```python
from build123d import *

# Parameters (mm, degrees)
BOSS_EXTRUDE1_DEPTH = 428


with BuildPart() as part:
    # Sketch1 → Boss-Extrude1 (new body)
    with BuildSketch(Plane(origin=(0, 0, 0), x_dir=(0, 0, -1), z_dir=(1, 0, 0))):
        with BuildLine():
            Line((-12.5, 11.5), (-12.5, 3))
            Line((-12.5, 3), (-10.5, 3))
            Line((-10.5, 3), (-10.5, 6))
            Line((-10.5, 6), (-9.535533906, 6))
            Line((-9.535533906, 6), (-6.5, 2.964466094))
            Line((-6.5, 2.964466094), (-6.5, -2.964466094))
            Line((-6.5, -2.964466094), (-9.535533906, -6))
            Line((-9.535533906, -6), (-10.5, -6))
            Line((-10.5, -6), (-10.5, -3))
            Line((-10.5, -3), (-12.5, -3))
            Line((-12.5, -3), (-12.5, -11.5))
            ThreePointArc((-12.5, -11.5), (-12.207106781, -12.207106781), (-11.5, -12.5))
            Line((-11.5, -12.5), (-3, -12.5))
            Line((-3, -12.5), (-3, -10.5))
            Line((-3, -10.5), (-6, -10.5))
            Line((-6, -10.5), (-6, -9.535533906))
            Line((-6, -9.535533906), (-2.964466094, -6.5))
            Line((-2.964466094, -6.5), (2.964466094, -6.5))
            Line((2.964466094, -6.5), (6, -9.535533906))
            Line((6, -9.535533906), (6, -10.5))
            Line((6, -10.5), (3, -10.5))
            Line((3, -10.5), (3, -12.5))
            Line((3, -12.5), (11.5, -12.5))
            ThreePointArc((11.5, -12.5), (12.207106781, -12.207106781), (12.5, -11.5))
            Line((12.5, -11.5), (12.5, -3))
            Line((12.5, -3), (10.5, -3))
            Line((10.5, -3), (10.5, -6))
            Line((10.5, -6), (9.535533906, -6))
            Line((9.535533906, -6), (6.5, -2.964466094))
            Line((6.5, -2.964466094), (6.5, 2.964466094))
            Line((6.5, 2.964466094), (9.535533906, 6))
            Line((9.535533906, 6), (10.5, 6))
            Line((10.5, 6), (10.5, 3))
            Line((10.5, 3), (12.5, 3))
            Line((12.5, 3), (12.5, 11.5))
            ThreePointArc((12.5, 11.5), (12.207106781, 12.207106781), (11.5, 12.5))
            Line((11.5, 12.5), (3, 12.5))
            Line((3, 12.5), (3, 10.5))
            Line((3, 10.5), (6, 10.5))
            Line((6, 10.5), (6, 9.535533906))
            Line((6, 9.535533906), (2.964466094, 6.5))
            Line((2.964466094, 6.5), (-2.964466094, 6.5))
            Line((-2.964466094, 6.5), (-6, 9.535533906))
            Line((-6, 9.535533906), (-6, 10.5))
            Line((-6, 10.5), (-3, 10.5))
            Line((-3, 10.5), (-3, 12.5))
            Line((-3, 12.5), (-11.5, 12.5))
            ThreePointArc((-11.5, 12.5), (-12.207106781, 12.207106781), (-12.5, 11.5))
        make_face()
        with BuildLine():
            Line((-3.087755464, -1.885673936), (-3.585519377, -2.383437849))
            ThreePointArc((-3.585519377, -2.383437849), (-4.599238816, -4.599238816), (-2.383437849, -3.585519377))
            Line((-2.383437849, -3.585519377), (-1.885673936, -3.087755464))
            ThreePointArc((-1.885673936, -3.087755464), (-1.720751743, -3.0036254), (-1.537849315, -3.032329053))
            ThreePointArc((-1.537849315, -3.032329053), (0, -3.4), (1.537849315, -3.032329053))
            ThreePointArc((1.537849315, -3.032329053), (1.720751743, -3.0036254), (1.885673936, -3.087755464))
            Line((1.885673936, -3.087755464), (2.383437849, -3.585519377))
            ThreePointArc((2.383437849, -3.585519377), (4.599238816, -4.599238816), (3.585519377, -2.383437849))
            Line((3.585519377, -2.383437849), (3.087755464, -1.885673936))
            ThreePointArc((3.087755464, -1.885673936), (3.0036254, -1.720751743), (3.032329053, -1.537849315))
            ThreePointArc((3.032329053, -1.537849315), (3.4, 0), (3.032329053, 1.537849315))
            ThreePointArc((3.032329053, 1.537849315), (3.0036254, 1.720751743), (3.087755464, 1.885673936))
            Line((3.087755464, 1.885673936), (3.585519377, 2.383437849))
            ThreePointArc((3.585519377, 2.383437849), (4.599238816, 4.599238816), (2.383437849, 3.585519377))
            Line((2.383437849, 3.585519377), (1.885673936, 3.087755464))
            ThreePointArc((1.885673936, 3.087755464), (1.720751743, 3.0036254), (1.537849315, 3.032329053))
            ThreePointArc((1.537849315, 3.032329053), (0, 3.4), (-1.537849315, 3.032329053))
            ThreePointArc((-1.537849315, 3.032329053), (-1.720751743, 3.0036254), (-1.885673936, 3.087755464))
            Line((-1.885673936, 3.087755464), (-2.383437849, 3.585519377))
            ThreePointArc((-2.383437849, 3.585519377), (-4.599238816, 4.599238816), (-3.585519377, 2.383437849))
            Line((-3.585519377, 2.383437849), (-3.087755464, 1.885673936))
            ThreePointArc((-3.087755464, 1.885673936), (-3.0036254, 1.720751743), (-3.032329053, 1.537849315))
            ThreePointArc((-3.032329053, 1.537849315), (-3.4, 0), (-3.032329053, -1.537849315))
            ThreePointArc((-3.032329053, -1.537849315), (-3.0036254, -1.720751743), (-3.087755464, -1.885673936))
        make_face(mode=Mode.SUBTRACT)
        with BuildLine():
            Line((-11.25, 9.75), (-11.25, 7.976197667))
            ThreePointArc((-11.25, 7.976197667), (-10.817878403, 7.329481994), (-10.055025253, 7.48122292))
            Line((-10.055025253, 7.48122292), (-9.475230868, 8.061017306))
            Line((-9.475230868, 8.061017306), (-8.768124087, 7.353910524))
            ThreePointArc((-8.768124087, 7.353910524), (-7.353910524, 7.353910524), (-7.353910524, 8.768124087))
            Line((-7.353910524, 8.768124087), (-8.061017306, 9.475230868))
            Line((-8.061017306, 9.475230868), (-7.48122292, 10.055025253))
            ThreePointArc((-7.48122292, 10.055025253), (-7.329481994, 10.817878403), (-7.976197667, 11.25))
            Line((-7.976197667, 11.25), (-9.75, 11.25))
            ThreePointArc((-9.75, 11.25), (-10.810660172, 10.810660172), (-11.25, 9.75))
        make_face(mode=Mode.SUBTRACT)
        with BuildLine():
            Line((8.061017306, 9.475230868), (7.353910524, 8.768124087))
            ThreePointArc((7.353910524, 8.768124087), (7.353910524, 7.353910524), (8.768124087, 7.353910524))
            Line((8.768124087, 7.353910524), (9.475230868, 8.061017306))
            Line((9.475230868, 8.061017306), (10.055025253, 7.48122292))
            ThreePointArc((10.055025253, 7.48122292), (10.817878403, 7.329481994), (11.25, 7.976197667))
            Line((11.25, 7.976197667), (11.25, 9.75))
            ThreePointArc((11.25, 9.75), (10.810660172, 10.810660172), (9.75, 11.25))
            Line((9.75, 11.25), (7.976197667, 11.25))
            ThreePointArc((7.976197667, 11.25), (7.329481994, 10.817878403), (7.48122292, 10.055025253))
            Line((7.48122292, 10.055025253), (8.061017306, 9.475230868))
        make_face(mode=Mode.SUBTRACT)
        with BuildLine():
            Line((-9.475230868, -8.061017306), (-10.055025253, -7.48122292))
            ThreePointArc((-10.055025253, -7.48122292), (-10.817878403, -7.329481994), (-11.25, -7.976197667))
            Line((-11.25, -7.976197667), (-11.25, -9.75))
            ThreePointArc((-11.25, -9.75), (-10.810660172, -10.810660172), (-9.75, -11.25))
            Line((-9.75, -11.25), (-7.976197667, -11.25))
            ThreePointArc((-7.976197667, -11.25), (-7.329481994, -10.817878403), (-7.48122292, -10.055025253))
            Line((-7.48122292, -10.055025253), (-8.061017306, -9.475230868))
            Line((-8.061017306, -9.475230868), (-7.353910524, -8.768124087))
            ThreePointArc((-7.353910524, -8.768124087), (-7.353910524, -7.353910524), (-8.768124087, -7.353910524))
            Line((-8.768124087, -7.353910524), (-9.475230868, -8.061017306))
        make_face(mode=Mode.SUBTRACT)
        with BuildLine():
            Line((9.475230868, -8.061017306), (8.768124087, -7.353910524))
            ThreePointArc((8.768124087, -7.353910524), (7.353910524, -7.353910524), (7.353910524, -8.768124087))
            Line((7.353910524, -8.768124087), (8.061017306, -9.475230868))
            Line((8.061017306, -9.475230868), (7.48122292, -10.055025253))
            ThreePointArc((7.48122292, -10.055025253), (7.329481994, -10.817878403), (7.976197667, -11.25))
            Line((7.976197667, -11.25), (9.75, -11.25))
            ThreePointArc((9.75, -11.25), (10.810660172, -10.810660172), (11.25, -9.75))
            Line((11.25, -9.75), (11.25, -7.976197667))
            ThreePointArc((11.25, -7.976197667), (10.817878403, -7.329481994), (10.055025253, -7.48122292))
            Line((10.055025253, -7.48122292), (9.475230868, -8.061017306))
        make_face(mode=Mode.SUBTRACT)
    extrude(amount=BOSS_EXTRUDE1_DEPTH)


solid = part.part
```
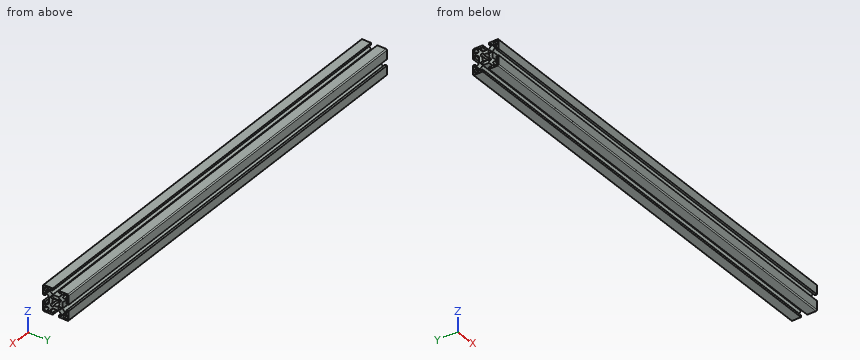
The listing builds one solid part. Answer for the finished solid, in the listing's coordinates (mm). Give positions to 0.01 mm unless a question says otherwise; leave off trailing zeros. Put each result on its own line as item: value. Start each with the question number.
Item 1: The part is cut by section A-A, the plane x = 237. State how many separate pieces and enclosed holes the cut face has, and give its area (3 significant figures).
Item 2: Find the intervals of material crossed by line 1 along Y through (x, z) = (275.5, -3.68); line 2 along Z through (x, y) = (67, 11); line 3 along Z through (x, y) = (325, 10), in increasing order.
Item 3: A flat-ended cylindrical pin translates along its axis: P1, Ø3, axis at x = 194.5, y = -0.5, coming from the -Z side. Find the tip coordinate at first contact, or state that the pin passes through.
Answer key:
1. separate pieces: 1
1. enclosed holes: 5
1. area: 302 mm²
2. line 1: y = -12.5 to -10.5, -7.22 to -4.98, -2.38 to 2.38, 4.98 to 7.22, 10.5 to 12.5
2. line 2: z = -12.5 to -10.58, -7.44 to -3, 3 to 7.44, 10.58 to 12.5
2. line 3: z = -12.5 to -11.23, -7.54 to -6, 6 to 7.54, 11.23 to 12.5
3. P1: stops at z = -6.5
